from build123d import *

# Parameters (mm, degrees)
SKETCH2_W               = 43.942
SKETCH2_H               = 127
BOSS_EXTRUDE1_DEPTH     = 6.35
M6_CLEARANCE_HOLE1_D    = 6.6
SKETCH5_W               = 7.0505
SKETCH5_H               = 127
CUT_EXTRUDE1_DEPTH      = 1
CUT_EXTRUDE1_DEPTH_BACK = 7.35
SKETCH6_W               = 27.8745
SKETCH6_H               = 3.175
CUT_EXTRUDE2_DEPTH      = 7.35
SKETCH7_W               = 6.35
SKETCH7_H               = 4.7625
CUT_EXTRUDE3_DEPTH      = 7.35
SKETCH8_R               = 3.3
CUT_EXTRUDE4_DEPTH      = 1
CUT_EXTRUDE4_DEPTH_BACK = 7.35


with BuildPart() as part:
    # Sketch2 → Boss-Extrude1 (new body)
    with BuildSketch(Plane.XY):
        with Locations((21.971, 63.5)):
            Rectangle(SKETCH2_W, SKETCH2_H)
    extrude(amount=BOSS_EXTRUDE1_DEPTH)

    # M6 Clearance Hole1 (through all)
    with Locations(Plane.XY.offset(6.35)):
        with Locations((17.4625, 31.75), (17.4625, 95.25)):
            Hole(M6_CLEARANCE_HOLE1_D / 2)

    # Sketch5 → Cut-Extrude1 (cut, two sides)
    with BuildSketch(Plane.XY.offset(6.35)) as cut_extrude1_sk:
        with Locations((3.52525, 63.5)):
            Rectangle(SKETCH5_W, SKETCH5_H)
    extrude(amount=CUT_EXTRUDE1_DEPTH, mode=Mode.SUBTRACT)
    extrude(cut_extrude1_sk.sketch, amount=-CUT_EXTRUDE1_DEPTH_BACK, mode=Mode.SUBTRACT)

    # Sketch6 → Cut-Extrude2 (cut, through all)
    with BuildSketch(Plane.XY.offset(6.35)):
        Polygon((7.0505, 123.825), (7.0505, 120.65), (37.30625, 120.65), (37.30625, 127), (34.925, 127), (34.925, 123.825), align=None)
        with Locations((20.98775, 125.4125)):
            Rectangle(SKETCH6_W, SKETCH6_H)
        Polygon((37.30625, 66.675), (7.0505, 66.675), (7.0505, 63.5), (34.925, 63.5), (34.925, 60.325), (7.0505, 60.325), (7.0505, 57.15), (37.30625, 57.15), align=None)
        with Locations((20.98775, 61.9125)):
            Rectangle(SKETCH6_W, SKETCH6_H)
        Polygon((37.30625, 0), (37.30625, 6.35), (7.0505, 6.35), (7.0505, 3.175), (34.925, 3.175), (34.925, 0), align=None)
        with Locations((20.98775, 1.5875)):
            Rectangle(SKETCH6_W, SKETCH6_H)
    extrude(amount=-CUT_EXTRUDE2_DEPTH, mode=Mode.SUBTRACT)

    # Sketch7 → Cut-Extrude3 (cut, through all)
    with BuildSketch(Plane.XY.offset(6.35)):
        with Locations((31.115, 118.26875)):
            Rectangle(SKETCH7_W, SKETCH7_H)
        with Locations((31.115, 69.05625)):
            Rectangle(SKETCH7_W, SKETCH7_H)
        with Locations((31.115, 54.76875)):
            Rectangle(SKETCH7_W, SKETCH7_H)
        with Locations((31.115, 8.73125)):
            Rectangle(SKETCH7_W, SKETCH7_H)
    extrude(amount=-CUT_EXTRUDE3_DEPTH, mode=Mode.SUBTRACT)

    # Sketch8 → Cut-Extrude4 (cut, two sides)
    with BuildSketch(Plane.XY.offset(6.35)) as cut_extrude4_sk:
        Polygon((37.30625, 66.675), (37.30625, 63.5), (43.942, 63.5), (43.942, 127), (37.30625, 127), (37.30625, 120.65), (34.29, 120.65), (34.29, 115.8875), (27.94, 115.8875), (27.94, 120.65), (7.0505, 120.65), (7.0505, 66.675), (27.94, 66.675), (27.94, 71.4375), (34.29, 71.4375), (34.29, 66.675), align=None)
        with Locations((17.4625, 95.25)):
            Circle(SKETCH8_R, mode=Mode.SUBTRACT)
    extrude(amount=CUT_EXTRUDE4_DEPTH, mode=Mode.SUBTRACT)
    extrude(cut_extrude4_sk.sketch, amount=-CUT_EXTRUDE4_DEPTH_BACK, mode=Mode.SUBTRACT)


solid = part.part
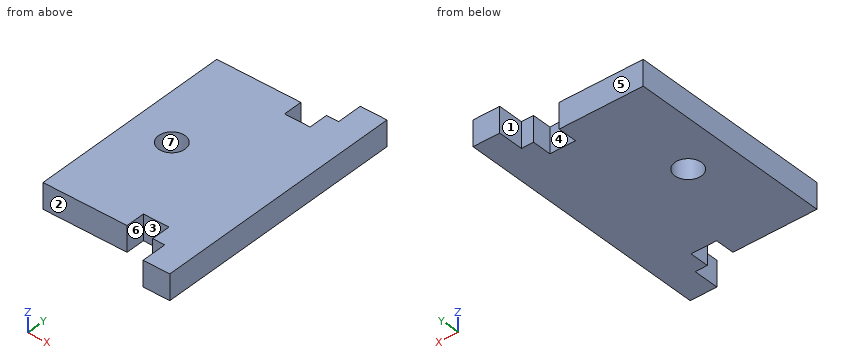
The listing builds one solid part. Answer for the finished solid, in the listing's coordinates (mm). Face numbers are marked on the shaded views. A direction names the side the tool comes from. Give positions to 0.01 mm unless a question says otherwise; leave off trailing zeros. Write each loop counter-clockwise with the first axis right and the second up, starting at its lowest first coordinate (ties: lowest second). Pieces come first, ordered by that corner, then holes. Notation, with made-up numbers: (-2.75, 26) -> (8.25, 26) arc R19 ccw to (8.25, 60) -> close; hole circle Ø8 at (47.5, 64). An arc over 180 degrees is marked (long way). One line per question, with ' | ' between items. Start each with the question number.
1. Find the intervals of material crossed by probe 1 along Y at (x, z) = (17.5, 5.75); probe 2 along X at (y, z) = (7, 2.25); probe 3 along Y at (x, z) = (9, 2), in increasing order.
2. Section B-B (y = 31.75) is taken. Determine the outline of the cut face in (x, z), plus the area to 3 significant figures.
3. Section A-A (z = 2.75) is taken. Determine the outline of the cut face in (x, y), plus the area to 3 significant figures.
4. Given pin 1 Ø3.5 at (x, z) = (35.5, 4.5) entering from -Y; pin 2 Ø3 at (y, z) = (61, 2.5) entering from -X; pin 3 Ø0.9 at (x, z) = (36.5, 3.5) entering from +Y, each flat-ended and moving along its own axis, determine where each tip first touches the part or whether it passes through.
5. Section C-C (x = 36.5) is taken. Determine the outline of the cut face in (y, z), plus the area to 3 significant figures.
6. For a pull along Y with two mould halves and no side action, classify the marked faces 5, 6 and 7 as pulls with the +Y half, pulls with the -Y half, needs draft (parallel to the pull), parting line crosses it, or undercut.
7. For the marked faces 1, 2, 3 and 4, determine the directions among +Z, -Z, +X, -X, +Y, -Y from which every point of the face is accessible in a straight line to the end or side of a thin tool.
Response values:
1) probe 1: 6.35 to 28.45, 35.05 to 57.15 | probe 2: 7.05 to 27.94, 34.29 to 43.94 | probe 3: 6.35 to 57.15
2) outline: (7.05, 0) -> (14.16, 0) -> (14.16, 6.35) -> (7.05, 6.35) -> close; (20.76, 0) -> (43.94, 0) -> (43.94, 6.35) -> (20.76, 6.35) -> close | area: 192 mm2
3) outline: (7.05, 6.35) -> (27.94, 6.35) -> (27.94, 11.11) -> (34.29, 11.11) -> (34.29, 6.35) -> (37.31, 6.35) -> (37.31, 0) -> (43.94, 0) -> (43.94, 63.5) -> (37.31, 63.5) -> (37.31, 57.15) -> (34.29, 57.15) -> (34.29, 52.39) -> (27.94, 52.39) -> (27.94, 57.15) -> (7.05, 57.15) -> close; hole circle Ø6.6 at (17.46, 31.75) | area: 1,860 mm2
4) pin 1: y = 6.35 | pin 2: x = 37.31 | pin 3: y = 57.15
5) outline: (6.35, 0) -> (57.15, 0) -> (57.15, 6.35) -> (6.35, 6.35) -> close | area: 323 mm2
6) face 5: pulls with the +Y half | face 6: needs draft | face 7: undercut
7) face 1: +Z, -Z, -X, +Y | face 2: +Z, -Z, -X, -Y | face 3: +Z, -Z, -Y | face 4: +Z, -Z, +Y
